Work out the finished part from the listing and answer in its coordinate system (mm). Face numbers are marked on the shaded views. A direction names the side the tool comes from. Give positions to 0.01 mm unless a question says otherwise; leave off trailing zeros. Order: outer loops, then holes, each group sorted by start corner. A loop starts at its lowest first (then second) coordinate and runs counter-clockwise, first axis right, second up.
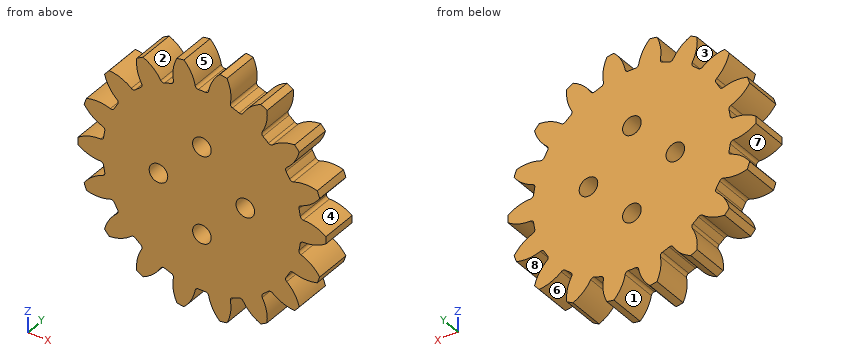
```python
from build123d import *

# Parameters (mm, degrees)
SKETCH_1_R               = 20
SKETCH_1_R_2             = 1.5
EXTRUDE_1_DEPTH          = 6
CUT_EXTRUDE_1_DEPTH      = 29.91366459
PATTERN_CIRCULAR_1_COUNT = 18


with BuildPart() as part:
    # 草图1 → 凸台-拉伸1 (new body)
    with BuildSketch(Plane(origin=(0, 0, 0), x_dir=(1, 0, 0), z_dir=(0, 1, 0))):
        with Locations(Location((0, 0, 0), (0, 0, 270))):
            Circle(SKETCH_1_R)
        with Locations(Location((0, 7, 0), (0, 0, 270))):
            Circle(SKETCH_1_R_2, mode=Mode.SUBTRACT)
        with Locations(Location((7, 0, 0), (0, 0, 270))):
            Circle(SKETCH_1_R_2, mode=Mode.SUBTRACT)
        with Locations(Location((0, -7, 0), (0, 0, 270))):
            Circle(SKETCH_1_R_2, mode=Mode.SUBTRACT)
        with Locations(Location((-7, 0, 0), (0, 0, 270))):
            Circle(SKETCH_1_R_2, mode=Mode.SUBTRACT)
    extrude(amount=EXTRUDE_1_DEPTH)

    # 草图2 → 切除-拉伸1 (cut, symmetric)
    with BuildSketch(Plane(origin=(0, 0, 0), x_dir=(1, 0, 0), z_dir=(0, 1, 0))):
        with BuildLine():
            ThreePointArc((2.90303546, 19.78818802), (0, 20), (-2.90303546, 19.78818802))
            ThreePointArc((-2.90303546, 19.78818802), (-1.72363994, 18.240586555), (-1.086139037, 16.402207735))
            ThreePointArc((-1.086139037, 16.402207735), (-0.908122705, 16.100478627), (-0.57579122, 15.989636158))
            ThreePointArc((-0.57579122, 15.989636158), (0, 16), (0.57579122, 15.989636158))
            ThreePointArc((0.57579122, 15.989636158), (0.908122705, 16.100478627), (1.086139037, 16.402207735))
            ThreePointArc((1.086139037, 16.402207735), (1.72363994, 18.240586555), (2.90303546, 19.78818802))
        make_face()
    cut_extrude_1 = extrude(amount=CUT_EXTRUDE_1_DEPTH, both=True, mode=Mode.SUBTRACT)

    # 阵列(圆周)1: 切除-拉伸1 ×18 about axis
    pattern_circular_1_axis = Axis((0, 0, 0), (0, 1, 0))
    for i in range(1, PATTERN_CIRCULAR_1_COUNT):
        add(cut_extrude_1.rotate(pattern_circular_1_axis, i * 360 / PATTERN_CIRCULAR_1_COUNT), mode=Mode.SUBTRACT)


solid = part.part
```
1. Straight lines are drawn through the part: probe 1 along X at (y, z) = (4.75, 0); probe 2 along X at (y, z) = (3.2, 16.5); probe 3 along Z at (x, y) = (14.5, 4.4). For each, find the intervals that lie inside material, in ascending order.
Findings below:
probe 1: x = -20 to -8.5, -5.5 to 5.5, 8.5 to 20
probe 2: x = -10.53 to -7.8, -4.67 to -1.1, 1.1 to 4.67, 7.8 to 10.53
probe 3: z = -13.25 to -10, -7.24 to 7.24, 10 to 13.25
2. Which of the six approach directions +Z, -Z, +X, -X, +Y, -Y give full straight-line access (tool end or side, diameter ignored) to the marked faces 4, 5, 6, 7 and 8?
Findings below:
face 4: +X, +Y, -Y
face 5: +Z, +Y, -Y
face 6: -Z, +Y, -Y
face 7: -X, +Y, -Y
face 8: +Y, -Y
3. The part is cut by section A-A (x = 0). Write down the section's boundary in (y, z), then the cut area to 3 significant figures.
Findings below:
outline: (0, -16) - (6, -16) - (6, -8.5) - (0, -8.5) - close; (0, -5.5) - (6, -5.5) - (6, 5.5) - (0, 5.5) - close; (0, 8.5) - (6, 8.5) - (6, 16) - (0, 16) - close
area: 156 mm2
4. The part is cut by section B-B (z = 0). Write down the section's boundary in (x, y), then the cut area to 3 significant figures.
Findings below:
outline: (-20, 0) - (-8.5, 0) - (-8.5, 6) - (-20, 6) - close; (-5.5, 0) - (5.5, 0) - (5.5, 6) - (-5.5, 6) - close; (8.5, 0) - (20, 0) - (20, 6) - (8.5, 6) - close
area: 204 mm2
5. The part is cut by section D-D (y = 1.2). State how many separate pieces and enclosed holes the cut face has, then the cut area to 3 significant figures.
Findings below:
separate pieces: 1
enclosed holes: 4
area: 985 mm2
6. The mould has two halves that part along Z. Classify the marked faces 1, 2 and 3: pulls with the +Z half, pulls with the -Z half, needs draft (parallel to the pull), parting line crosses it, or undercut.
Findings below:
face 1: pulls with the -Z half
face 2: pulls with the +Z half
face 3: undercut
7. Given P1, Ø2, axis at x = -13.5, y = 4.5, coming from the +Z side; P2, Ø1.5, axis at x = -8.5, y = 1.5, coming from the +Z side, each flat-ended and moving along its own axis, determine where each tip first touches the part or whether it passes through.
Findings below:
P1: stops at z = 13.25
P2: stops at z = 17.49
8. The part is cut by section C-C (x = 7.5). Write down the section's boundary in (y, z), then the cut area to 3 significant figures.
Findings below:
outline: (0, -16.2) - (6, -16.2) - (6, -1.41) - (0, -1.41) - close; (0, 1.41) - (6, 1.41) - (6, 16.2) - (0, 16.2) - close
area: 177 mm2
